```python
from build123d import *

# Parameters (mm, degrees)
BOSS_EXTRUDE1_DEPTH     = 6.35
CHAMFER1_SIZE           = 3.175
CUT_EXTRUDE1_DEPTH      = 316.484
CUT_EXTRUDE1_DEPTH_BACK = 13.716
SKETCH2_R               = 50.8


with BuildPart() as part:
    # Sketch1 → Boss-Extrude1 (new body)
    with BuildSketch(Plane.XY):
        Polygon((254, 139.7), (0, 0), (254, 0), align=None)
        Polygon((254, 139.7), (254, 0), (304.8, 0), (330.2, 139.7), align=None)
    extrude(amount=BOSS_EXTRUDE1_DEPTH)

    # Chamfer1
    chamfer1_edges = [part.edges().sort_by_distance(p)[0] for p in [
        (317.5, 69.85, 0),
        (317.5, 69.85, 6.35),
        (127, 69.85, 6.35),
        (127, 69.85, 0),
    ]]
    chamfer(chamfer1_edges, length=CHAMFER1_SIZE - 0.0001)  # a hair under: the kernel refuses the full size

    # Sketch2 → Cut-Extrude1 (cut, two sides: drawn at the far end of the back side and taken through both)
    with BuildSketch(Plane(origin=(0, 0, 0), x_dir=(0, 0, -1), z_dir=(1, 0, 0)).offset(-CUT_EXTRUDE1_DEPTH_BACK)):
        with Locations((-3.175, -50.700684167)):
            Circle(SKETCH2_R)
    extrude(amount=CUT_EXTRUDE1_DEPTH + CUT_EXTRUDE1_DEPTH_BACK, mode=Mode.SUBTRACT)


solid = part.part
```
Source: CAD feature listing. Evaluate the final solid. Frame: model axes, mm. Round coordinates to 2 decimals unless told otherwise and drop trailing zeros. Order: outer loops, then holes, each group sorted by start corner. A loop starts at its lowest first (then second) coordinate and runs counter-clockwise, first axis right, second up. Notation, with made-up numbers: (-34.5, 75.5) -> (24.5, 75.5) arc R17 ccw to (24.5, 79.5) -> close; hole circle Ø9 at (-21, 18.25). An arc over 180 degrees is marked (long way). Use CSV: the item, a comma, the result in double quotes.
(1) Ray query, L1, parallel to Y at x = 267, z = 0.75; L2, parallel to Y at x = 289.5, z = 5; L3, parallel to X at y = 74.5, z = 6. Return the intervals inside material, ascending.
Report:
L1,"0.04 to 139.7"
L2,"0.07 to 139.7"
L3,"141.32 to 315.47"
(2) Section C-C on z = 1.75. Return the cut outline in (x, y).
Report:
outline,"(3.1, 0.08) -> (303.37, 0.08) -> (328.75, 139.7) -> (256.96, 139.7) -> close"
(3) First-contact query: pin 1 Ø1.5 at (x, z) = (72, 1.5) entering from +Y. Flat tip, straight axial feed; report the tip coordinate or a pass-through.
Report:
pin 1,"y = 38.64"
